Build history of the part. All positions in model axes, mm. Round coordinates to 2 decimals unless told otherwise and drop trailing zeros. Write each loop counter-clockwise with the first axis right and the second up, starting at its lowest first coordinate (ties: lowest second). Pieces come first, ordered by that corner, then holes. Notation, with made-up numbers: (-35.5, 40.25) - (-29.5, 40.25) arc R30 cw to (-29.5, 65.25) - close; hole circle Ø4 at (2, 62). An arc over 180 degrees is marked (long way). One line per question, with ' | ' between items.
from build123d import *

# Parameters (mm, degrees)
SKETCH1_W                 = 127
SKETCH1_H                 = 101.6
BOSS_EXTRUDE1_DEPTH       = 3.175
SKETCH2_W                 = 25.4
SKETCH2_H                 = 3.175
CUT_EXTRUDE1_DEPTH        = 6.35
LPATTERN1_COUNT           = 3
LPATTERN1_PITCH           = 50.8
CUT_EXTRUDE4_DEPTH        = 6.35
SKETCH8_W                 = 3.175
SKETCH8_H                 = 25.4
CUT_EXTRUDE6_DEPTH        = 6.35
SKETCH9_W                 = 25.4
SKETCH9_H                 = 3.175
CUT_EXTRUDE7_DEPTH        = 6.35
LPATTERN6_COUNT           = 2
LPATTERN6_PITCH           = 50.8
SKETCH16_W                = 4.3942
SKETCH16_H                = 17.145
SKETCH16_W_2              = 8.89
SKETCH16_H_2              = 3.302
CUT_EXTRUDE14_DEPTH       = 6.35
F_8_CLEARANCE_HOLE1_D     = 4.4958
F_8_CLEARANCE_HOLE1_DEPTH = 10.16
F_8_CLEARANCE_HOLE1_TIP   = 1.350674586
SKETCH20_R                = 1.75
CUT_EXTRUDE16_DEPTH       = 7.62
SKETCH25_W                = 25.4
SKETCH25_H                = 25.4
CUT_EXTRUDE20_DEPTH       = 7.62
F_4_CLEARANCE_HOLE1_D     = 3.2639
F_4_CLEARANCE_HOLE1_DEPTH = 10.16
F_4_CLEARANCE_HOLE1_TIP   = 0.980574487


with BuildPart() as part:
    # Sketch1 → Boss-Extrude1 (new body)
    with BuildSketch(Plane(origin=(0, 0, 0), x_dir=(0, 0, -1), z_dir=(1, 0, 0))):
        Rectangle(SKETCH1_W, SKETCH1_H)
    extrude(amount=BOSS_EXTRUDE1_DEPTH)

    # Sketch2 → Cut-Extrude1 (cut)
    with BuildSketch(Plane(origin=(3.175, 0, 0), x_dir=(0, 0, -1), z_dir=(1, 0, 0))):
        with Locations((-50.8, 49.2125)):
            Rectangle(SKETCH2_W, SKETCH2_H)
    cut_extrude1 = extrude(amount=-CUT_EXTRUDE1_DEPTH, mode=Mode.SUBTRACT)

    # LPattern1: Cut-Extrude1 ×3
    with Locations(*[(0, 0, -i * LPATTERN1_PITCH) for i in range(1, LPATTERN1_COUNT)]):
        add(cut_extrude1, mode=Mode.SUBTRACT)

    # Sketch5 → Cut-Extrude4 (cut)
    with BuildSketch(Plane(origin=(3.175, 0, 0), x_dir=(0, 0, -1), z_dir=(1, 0, 0))):
        with BuildLine():
            Line((-38.1, -38.1), (38.1, -38.1))
            ThreePointArc((38.1, -38.1), (50.8, -50.8), (38.1, -63.5))
            Line((38.1, -63.5), (-38.1, -63.5))
            ThreePointArc((-38.1, -63.5), (-50.8, -50.8), (-38.1, -38.1))
        make_face()
    extrude(amount=-CUT_EXTRUDE4_DEPTH, mode=Mode.SUBTRACT)

    # Sketch8 → Cut-Extrude6 (cut)
    with BuildSketch(Plane(origin=(3.175, 0, 0), x_dir=(0, 0, -1), z_dir=(1, 0, 0))):
        with Locations((61.9125, 12.7)):
            Rectangle(SKETCH8_W, SKETCH8_H)
    cut_extrude6 = extrude(amount=-CUT_EXTRUDE6_DEPTH, mode=Mode.SUBTRACT)

    # Sketch9 → Cut-Extrude7 (cut)
    with BuildSketch(Plane.ZY):
        with Locations((-25.4, -20.6375)):
            Rectangle(SKETCH9_W, SKETCH9_H)
    cut_extrude7 = extrude(amount=-CUT_EXTRUDE7_DEPTH, mode=Mode.SUBTRACT)

    # LPattern6: Cut-Extrude7 ×2
    with Locations(*[(0, 0, i * LPATTERN6_PITCH) for i in range(1, LPATTERN6_COUNT)]):
        add(cut_extrude7, mode=Mode.SUBTRACT)

    # Sketch16 → Cut-Extrude14 (cut)
    with BuildSketch(Plane.ZY):
        with Locations((0, 39.0525)):
            Rectangle(SKETCH16_W, SKETCH16_H)
        with Locations((0, 41.275)):
            Rectangle(SKETCH16_W_2, SKETCH16_H_2)
    extrude(amount=-CUT_EXTRUDE14_DEPTH, mode=Mode.SUBTRACT)

    # #8 Clearance Hole1
    with Locations(Plane.ZY):
        with Locations((0, -20.6375)):
            Hole(F_8_CLEARANCE_HOLE1_D / 2, depth=F_8_CLEARANCE_HOLE1_DEPTH)
            with Locations((0, 0, -(F_8_CLEARANCE_HOLE1_DEPTH + F_8_CLEARANCE_HOLE1_TIP / 2))):  # 118° drill point
                Cone(0, F_8_CLEARANCE_HOLE1_D / 2, F_8_CLEARANCE_HOLE1_TIP, mode=Mode.SUBTRACT)

    # Sketch20 → Cut-Extrude16 (cut)
    with BuildSketch(Plane.ZY):
        with Locations((-45.0725, 12.7)):
            Circle(SKETCH20_R)
        with Locations((-5.0725, 12.7)):
            Circle(SKETCH20_R)
        with BuildLine():
            Line((-35.3225, 23.6601), (-15.4775, 23.6601))
            ThreePointArc((-15.4775, 23.6601), (-11.941966094, 22.195633906), (-10.4775, 18.6601))
            Line((-10.4775, 18.6601), (-10.4775, 6.7399))
            ThreePointArc((-10.4775, 6.7399), (-11.941966094, 3.204366094), (-15.4775, 1.7399))
            Line((-15.4775, 1.7399), (-35.3225, 1.7399))
            ThreePointArc((-35.3225, 1.7399), (-38.858033906, 3.204366094), (-40.3225, 6.7399))
            Line((-40.3225, 6.7399), (-40.3225, 18.6601))
            ThreePointArc((-40.3225, 18.6601), (-38.858033906, 22.195633906), (-35.3225, 23.6601))
        make_face()
    extrude(amount=-CUT_EXTRUDE16_DEPTH, mode=Mode.SUBTRACT)

    # Sketch25 → Cut-Extrude20 (cut)
    with BuildSketch(Plane.ZY):
        with Locations((25.4, 12.7)):
            Rectangle(SKETCH25_W, SKETCH25_H)
    extrude(amount=-CUT_EXTRUDE20_DEPTH, mode=Mode.SUBTRACT)

    # Mirror3: Cut-Extrude6 across plane
    add(cut_extrude6.mirror(Plane.XY), mode=Mode.SUBTRACT)

    # #4 Clearance Hole1
    with Locations(Plane(origin=(3.175, 0, 0), x_dir=(0, 0, -1), z_dir=(1, 0, 0))):
        with Locations((-44.45, 12.7), (-6.35, 12.7)):
            Hole(F_4_CLEARANCE_HOLE1_D / 2, depth=F_4_CLEARANCE_HOLE1_DEPTH)
            with Locations((0, 0, -(F_4_CLEARANCE_HOLE1_DEPTH + F_4_CLEARANCE_HOLE1_TIP / 2))):  # 118° drill point
                Cone(0, F_4_CLEARANCE_HOLE1_D / 2, F_4_CLEARANCE_HOLE1_TIP, mode=Mode.SUBTRACT)


solid = part.part
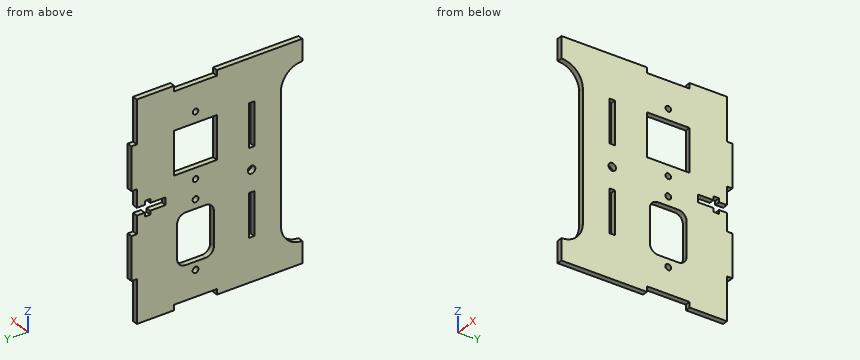
Q1. Saw through at B-B, the plane y = 12.7. List the corners of the cut face in (x, z) (1 decimal), then the cut area to 3 significant figures.
Found:
outline: (0, -60.3) - (3.2, -60.3) - (3.2, -46.8) - (0, -46.8) - close; (0, -43.3) - (3.2, -43.3) - (3.2, -40.3) - (0, -40.3) - close; (0, -10.5) - (3.2, -10.5) - (3.2, -6.8) - (0, -6.8) - close; (0, -3.3) - (3.2, -3.3) - (3.2, 4.7) - (0, 4.7) - close; (0, 8) - (3.2, 8) - (3.2, 12.7) - (0, 12.7) - close; (0, 38.1) - (3.2, 38.1) - (3.2, 42.8) - (0, 42.8) - close; (0, 46.1) - (3.2, 46.1) - (3.2, 60.3) - (0, 60.3) - close | area: 165 mm^2
Q2. Drop flat-ended pins along their axis: pin 1 (4 mm diameter, centred on y = -17, z = 34, fed in from -X); pin 2 (1 mm diameter, centred on x = 1.5, z = 8.5, fed in from +Y) (3 decimals); pin 3 (1.6 mm diameter, centred on x = 2.5, z = 21, fed in from -Y); pin 4 (1 mm diameter, centred on x = 2, y = 17.5, fed in from +Z) (3 decimals). Give the stop position or say it passes through.
Found:
pin 1: x = 0 | pin 2: y = 47.625 | pin 3: y = -38.1 | pin 4: z = 60.325
Q3. Saw through at C-C, the plane z = 31. List the corners of the cut face in (x, y) (3 decimals).
Found:
outline: (0, -38.1) - (3.175, -38.1) - (3.175, -22.225) - (0, -22.225) - close; (0, -19.05) - (3.175, -19.05) - (3.175, 0) - (0, 0) - close; (0, 25.4) - (3.175, 25.4) - (3.175, 50.8) - (0, 50.8) - close
Q4. Drill centre lines: L1, parallel to Y at x = 1.75, z = -33 (3 decimals); L2, parallel to Z at x = 2.75, y = -21; L3, parallel to Z at x = 2.05, y = 17.5 (1 decimal). Where is each one in solid material? Low to high. Write a range as from..to.
Found:
L1: -38.1..-22.225, -19.05..1.74, 23.66..50.8 | L2: -63.5..-38.1, -12.7..-2.22, 2.22..12.7, 38.1..63.5 | L3: -60.3..-40.3, -10.5..12.7, 38.1..60.3
Q5. Saw through at A-A, the plane z = 0. List the corners of the cut face in (x, y) (3 decimals), then the cut area to 3 significant figures.
Found:
outline: (0, -38.1) - (3.175, -38.1) - (3.175, -22.885) - (0, -22.885) - close; (0, -18.39) - (3.175, -18.39) - (3.175, 30.48) - (0, 30.48) - close | area: 203 mm^2
Q6. Saw through at D-D, the plane y = -42.5. List the corners of the cut face in (x, z) (1 decimal), then the cut area to 3 significant figures.
Found:
outline: (0, -63.5) - (3.2, -63.5) - (3.2, -47.7) - (0, -47.7) - close; (0, 47.7) - (3.2, 47.7) - (3.2, 63.5) - (0, 63.5) - close | area: 100 mm^2
